Input: part model. Units: mm. Frame: model coordinates. Face numbers are marked on the shaded views. Round coordinates to 2 decimals unless told otherwise and drop trailing zeros. Loops run counter-clockwise (first coordinate to the right, second up) from the corner with the lowest first, then second, coordinate; pieces in that order, holes last. Notation, with made-up numbers: M 15,-20.5 L 46,-20.5 A26 cw 46,11.5 Z; hole C 62,9.25 d5. An arc over 180 degrees is marked long. Use one line per item in the form item = value. Start each with the question number.
Q1. First-contact query: P1, Ø6, axis at y = -37, z = 37.5, coming from the +X side; P2, Ø2, axis at y = -47, z = 16.5, coming from the -X side; P3, Ø12.5, axis at x = -18.75, z = 32.476, coming from the +Y side; P4, Ø12, axis at x = 12.5, y = -95.5, coming from the +Z side. Flat tips, straight axial feed; report the tip coordinate or a pass-through.
Q2. Mould query, pull axis Z, two halves, no side actions, for the marked faces 1, 2, 3 and 4. Classes: pulls with the +Z half, pulls with the -Z half, needs draft (parallel to the pull), parting line crosses it, or undercut.
Q3. Section query A-A, the plane z = 30.5. Output: boundary loops of the cut face in (x, y).
Q4. Section query C-C, the plane y = -55. State how many separate pieces and enclosed holes the cut face has, and give its area (3 significant figures).
Q5. Ray query, line 1 along X through (y, z) = (-80, 57); line 2 along X through (y, z) = (-100, 52.5); line 3 along Z through (x, y) = (17, -54.5). Return the intervals inside material, ascending.
Q6. Section query B-B, the plane z = 17. Output: boundary loops of the cut face in (x, y).
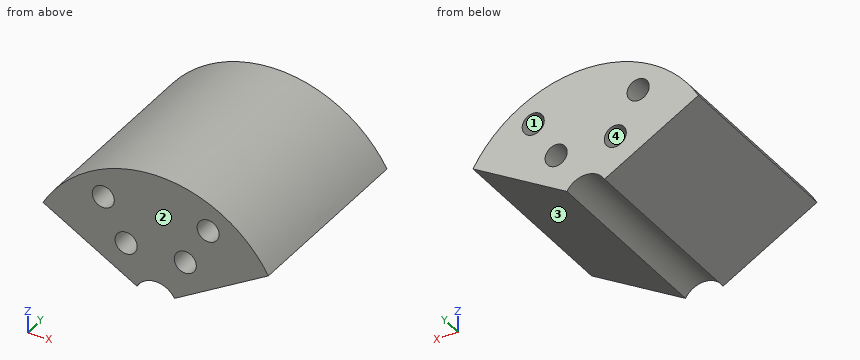
```python
from build123d import *

# Parameters (mm, degrees)
F_3DSKETCH2_R  = 6.999845998
EXTRUDE3_DEPTH = 124.992


with BuildPart() as part:
    # 3DSketch2 → Extrude3 (new body)
    with BuildSketch(Plane(origin=(-18.75, -123.736, 32.476), x_dir=(0.8870183146835777, -1.4196355069849515e-13, 0.4617342411126832), z_dir=(0, -1, 0))):
        with BuildLine():
            Line((84.057647161, -33.864344653), (15.373349185, -36.864404238))
            add(Edge.make_bspline(
                [(15.373349185, -36.864404238), (15.352068384, -36.534110534), (15.309494256, -35.873328697), (15.15380243, -34.89161264), (14.935730394, -33.922345945), (14.643794083, -32.972322164), (14.286702831, -32.044997482), (13.863035519, -31.145928893), (13.374501259, -30.280509448), (12.825956594, -29.451879273), (12.217498956, -28.666136437), (11.555519853, -27.925462519), (10.84179713, -27.234048158), (10.079158018, -26.597430452), (9.273057277, -26.016087573), (8.427361578, -25.494638196), (7.545715962, -25.035700694), (6.633485756, -24.64206797), (5.694906567, -24.315223891), (4.735979636, -24.055686494), (3.760225519, -23.867649672), (2.773801545, -23.750253207), (1.781160185, -23.702549632), (0.787754631, -23.728523084), (-0.2013641, -23.8247555), (-1.180838094, -23.993423853), (-2.145269372, -24.232834664), (-3.090921175, -24.538636337), (-4.009966724, -24.915980503), (-4.903428486, -25.351563375), (-5.469117643, -25.695715914), (-5.751878998, -25.867741552)],
                knots=[0, 0, 0, 0, 0.034470888, 0.068962068, 0.103436508, 0.137919118, 0.17241911, 0.20689509, 0.241383087, 0.275880421, 0.310348632, 0.344841071, 0.379302859, 0.41379577, 0.448262511, 0.482772834, 0.517227166, 0.551737489, 0.58620423, 0.620697141, 0.655158929, 0.689651368, 0.724119579, 0.758616913, 0.79310491, 0.82758089, 0.862080882, 0.896563492, 0.931037932, 0.965529112, 1, 1, 1, 1], degree=3))
            Line((-5.751878998, -25.867741552), (-42.691947897, 32.114707997))
            add(Edge.make_bspline(
                [(84.057647161, -33.864344653), (83.929496966, -31.881927263), (83.673219895, -27.917453198), (82.746706821, -22.024979481), (81.427672342, -16.211783357), (79.684589433, -10.509460987), (77.535515525, -4.948506144), (74.991650083, 0.443580722), (72.065661239, 5.63846846), (68.77170116, 10.608095708), (65.128087834, 15.327241456), (61.152593676, 19.770248775), (56.867676078, 23.91550345), (52.295461541, 27.741669794), (47.45762087, 31.226291453), (42.381892258, 34.353953282), (37.093279559, 37.106921885), (31.61985405, 39.47058486), (25.990484034, 41.43463264), (20.233707282, 42.985186118), (14.380348982, 44.117375042), (8.460577738, 44.825313071), (2.504980102, 45.10300258), (-3.455233166, 44.950602481), (-9.38889544, 44.367574744), (-15.264902994, 43.358422936), (-21.052782359, 41.929020999), (-26.723582946, 40.085969417), (-32.241968491, 37.831968062), (-37.600141517, 35.210965428), (-40.994576154, 33.14685641), (-42.691947897, 32.114707997)],
                knots=[0, 0, 0, 0, 0.034483919, 0.068961564, 0.103450466, 0.137933366, 0.172414368, 0.206896206, 0.241380972, 0.27586552, 0.310346021, 0.3448291, 0.379311579, 0.413791406, 0.448274645, 0.482761184, 0.517238816, 0.551725355, 0.586208594, 0.620688421, 0.6551709, 0.689653979, 0.72413448, 0.758619028, 0.793103794, 0.827585632, 0.862066634, 0.896549534, 0.931038436, 0.965516081, 1, 1, 1, 1], degree=3))
        make_face()
        with Locations(Location((0, 0, 0), (0, 0, 152.500928353))):
            Circle(F_3DSKETCH2_R, mode=Mode.SUBTRACT)
        with Locations(Location((-1.265310097, 28.972611469, 0), (0, 0, 152.500928353))):
            Circle(F_3DSKETCH2_R, mode=Mode.SUBTRACT)
        with Locations(Location((33.263186801, -17.315034042, 0), (0, 0, 152.500928353))):
            Circle(F_3DSKETCH2_R, mode=Mode.SUBTRACT)
        with Locations(Location((57.721407829, -1.732715565, 0), (0, 0, 152.500928353))):
            Circle(F_3DSKETCH2_R, mode=Mode.SUBTRACT)
    extrude(amount=-EXTRUDE3_DEPTH)


solid = part.part
```
Results found:
q1.P1 = 70.15
q1.P2 = -30.31
q1.P3 = through
q1.P4 = 82.24
q2.face_1 = undercut
q2.face_2 = needs draft
q2.face_3 = pulls with the -Z half
q2.face_4 = undercut
q3.outline = M -52.83,-123.74 L -25.47,-123.74 L -25.47,1.26 L -52.83,1.26 Z; M -12.03,-123.74 L 12.03,-123.74 L 12.03,1.26 L -12.03,1.26 Z; M 25.47,-123.74 L 52.83,-123.74 L 52.83,1.26 L 25.47,1.26 Z
q4.separate_pieces = 1
q4.enclosed_holes = 4
q4.area = 6,310 mm²
q5.line_1 = -59.64 to -40.22, -26.28 to 26.28, 40.22 to 59.64
q5.line_2 = -63.64 to -38.05, -28.45 to 28.45, 38.05 to 63.64
q5.line_3 = 9.81 to 25.7, 39.25 to 80.73
q6.outline = M -29.44,-123.74 L 29.44,-123.74 L 29.44,1.26 L -29.44,1.26 Z
